Can you work these out from the model? Positions are in its coordinate system, mm. Face numbers are marked on the shaded views. A direction names the side the tool comes from. Coordinates: 2 decimals unless noted, no trailing zeros. Order: outer loops, then holes, each group sorted by start corner. A loop starts at its lowest first (then second) coordinate and runs counter-clockwise, first axis right, second up. Notation, with made-up numbers: M 63,69 L 83,69 A10 ccw 83,73 Z; hole C 43,42.25 d2. An arc over 180 degrees is marked long. Answer as a JSON object with one key per item and string values.
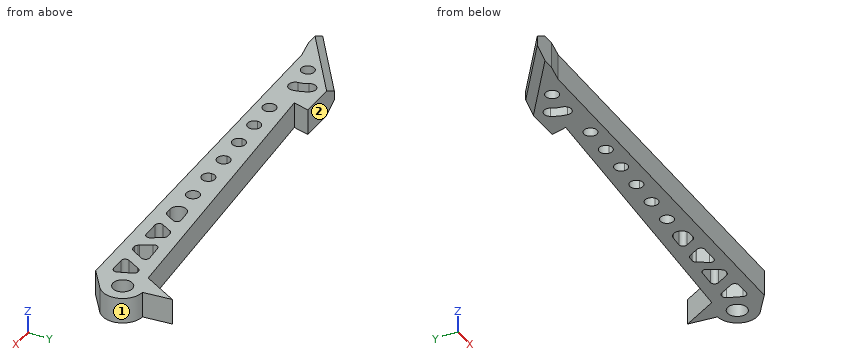
from build123d import *

# Parameters (mm, degrees)
SKETCH1_R           = 3.2639
SKETCH1_R_2         = 4.8025
BOSS_EXTRUDE1_DEPTH = 12.7
EXTRUDE_THIN1_DEPTH = 12.7
FILLET1_R           = 2
SKETCH3_R           = 3.2639
CUT_EXTRUDE1_DEPTH  = 222.669325799
CHAMFER1_SIZE       = 4


with BuildPart() as part:
    # Sketch1 → Boss-Extrude1 (new body)
    with BuildSketch(Plane.XY):
        with BuildLine():
            Line((-220, -20.475), (-207.3, -20.475))
            Line((-207.3, -20.475), (-197.3, -18.475))
            Line((-197.3, -18.475), (-5, -15.975))
            Line((-5, -15.975), (5.868885021, -8.096677628))
            ThreePointArc((5.868885021, -8.096677628), (9.584297561, 2.85328587), (0.484930071, 9.988235221))
            Line((0.484930071, 9.988235221), (-0.740940503, 24))
            Line((-0.740940503, 24), (-10.691733631, 6.764720727))
            Line((-10.691733631, 6.764720727), (-162.296299831, -3.282137227))
            Line((-162.296299831, -3.282137227), (-160.296299831, 4.525))
            Line((-160.296299831, 4.525), (-184.296299831, 4.525))
            Line((-184.296299831, 4.525), (-220, -20.475))
        make_face()
        with Locations((-154, -10.975)):
            Circle(SKETCH1_R, mode=Mode.SUBTRACT)
        with BuildLine():
            ThreePointArc((-135.489653222, -10.110575335), (-138.597743308, -13.523178805), (-142.010346778, -10.415088719))
            ThreePointArc((-142.010346778, -10.415088719), (-138.902256692, -7.00248525), (-135.489653222, -10.110575335))
        make_face(mode=Mode.SUBTRACT)
        with BuildLine():
            ThreePointArc((-120.239653222, -9.398407362), (-123.347743308, -12.811010832), (-126.760346778, -9.702920746))
            ThreePointArc((-126.760346778, -9.702920746), (-123.652256692, -6.290317277), (-120.239653222, -9.398407362))
        make_face(mode=Mode.SUBTRACT)
        with BuildLine():
            ThreePointArc((-104.989653222, -8.686239389), (-108.097743308, -12.098842859), (-111.510346778, -8.990752773))
            ThreePointArc((-111.510346778, -8.990752773), (-108.402256692, -5.578149304), (-104.989653222, -8.686239389))
        make_face(mode=Mode.SUBTRACT)
        with BuildLine():
            ThreePointArc((-89.739653222, -7.974071416), (-92.847743308, -11.386674886), (-96.260346778, -8.2785848))
            ThreePointArc((-96.260346778, -8.2785848), (-93.152256692, -4.865981331), (-89.739653222, -7.974071416))
        make_face(mode=Mode.SUBTRACT)
        with Locations((-77.75, -7.414160135)):
            Circle(SKETCH1_R, mode=Mode.SUBTRACT)
        with BuildLine():
            ThreePointArc((-63.032372648, -10.728944003), (-67.081236547, -6.887586999), (-63.348870778, -2.738036629))
            Line((-63.348870778, -2.738036629), (-11.492502478, 0.698492886))
            Line((-11.492502478, 0.698492886), (-7.437965658, -10.006187802))
            Line((-7.437965658, -10.006187802), (-63.032372648, -10.728944003))
        make_face(mode=Mode.SUBTRACT)
        Circle(SKETCH1_R_2, mode=Mode.SUBTRACT)
    extrude(amount=BOSS_EXTRUDE1_DEPTH)

    # Sketch2 → Extrude-Thin1 (add)
    with BuildSketch(Plane.XY.offset(12.7)):
        Polygon((-18.82367626, 4.244152852), (-20.32367626, 1.646076641), (-26.38156986, -8.846502861), (-27.88156986, -11.444579073), (-23.11843014, -14.194579073), (-21.61843014, -11.596502861), (-15.560536539, -1.103923359), (-14.060536539, 1.494152852), align=None)
        Polygon((-29.564922949, -12.326360556), (-31.654014309, -8.915246766), (-37.279649193, 0.270412174), (-39.368740553, 3.681525964), (-44.059022015, 0.809025344), (-41.969930654, -2.602088446), (-36.34429577, -11.787747387), (-34.25520441, -15.198861177), align=None)
        Polygon((-51.506359784, 2.078266381), (-53.006359784, -0.51980983), (-58.05148802, -9.258228266), (-59.55148802, -11.856304478), (-54.7883483, -14.606304478), (-53.2883483, -12.008228266), (-48.243220063, -3.26980983), (-46.743220063, -0.671733619), align=None)
    extrude(amount=-EXTRUDE_THIN1_DEPTH)

    # Fillet1
    fillet1_edges = [part.edges().sort_by_distance(p)[0] for p in [
        (-37.198435549, -10.393089387, 6.35),
        (-42.723767146, -1.371207834, 6.35),
        (-30.79987453, -10.309904766, 6.35),
        (-36.525812701, -0.960468438, 6.35),
        (-58.869359177, -10.674822663, 6.35),
        (-53.926545163, -2.113617659, 6.35),
        (-52.470477143, -10.591633869, 6.35),
        (-47.323034685, -1.676002002, 6.35),
        (-7.437965658, -10.006187802, 6.35),
        (-11.492502478, 0.698492886, 6.35),
        (-14.640351161, 0.489884469, 6.35),
        (-21.243861639, 0.052268813, 6.35),
        (-27.199441017, -10.263097258, 6.35),
        (-20.800558983, -10.179908464, 6.35),
    ]]
    fillet(fillet1_edges, radius=FILLET1_R)

    # Sketch3 → Cut-Extrude1 (cut, through all)
    with BuildSketch(Plane.XY.offset(12.7)):
        with Locations((-188, -10.475)):
            Circle(SKETCH3_R)
        with BuildLine():
            ThreePointArc((-170.811018785, -8.85662125), (-171.599559812, -5.080022092), (-173.207049233, -1.57281866))
            ThreePointArc((-173.207049233, -1.57281866), (-177.688057419, -0.458809846), (-178.802066233, -4.939818032))
            ThreePointArc((-178.802066233, -4.939818032), (-177.802564412, -7.120520542), (-177.31226682, -9.468727432))
            ThreePointArc((-177.31226682, -9.468727432), (-173.755589711, -12.413298359), (-170.811018785, -8.85662125))
        make_face()
    extrude(amount=-CUT_EXTRUDE1_DEPTH, mode=Mode.SUBTRACT)

    # Chamfer1
    chamfer1_edges = [part.edges().sort_by_distance(p)[0] for p in [
        (-202.148149916, -7.975, 0),
        (-202.148149916, -7.975, 12.7),
    ]]
    chamfer(chamfer1_edges, length=CHAMFER1_SIZE)


solid = part.part
Item 1: Please list where these lines run through material, in increasing order: line 1 (Y direction, x = -188, z = 5.75); line 2 (Y direction, x = -154, z = 5.5); line 3 (Y direction, x = -205.5, z = 3) (3 decimals).
Answers follow:
{"line 1": "y = -18.35 to -13.74, -7.21 to 1.93", "line 2": "y = -17.91 to -14.24, -7.71 to -2.73", "line 3": "y = -20.115 to -11.543"}
Item 2: I want a section at B-B, the plane y = 14. Write out the boundary of the cut face in (x, z).
Answers follow:
{"outline": "M -6.51,0 L 0.13,0 L 0.13,12.7 L -6.51,12.7 Z"}
Item 3: I want a section at D-D, the plane z = 2. Give the number of separate pieces and of enclosed holes in the cut face, plus the area to 3 significant figures.
Answers follow:
{"separate pieces": "1", "enclosed holes": "13", "area": "3,460 mm^2"}
Item 4: I'm going to push flat-ended pins straight in: pin 1 (12.5 mm diameter, centred on x = 0, y = 0, fed in from +Z); pin 2 (1 mm diameter, centred on y = 15, z = 8.5, fed in from -X); pin 3 (3 mm diameter, centred on y = 15.5, z = 6, fed in from -X); pin 4 (5 mm diameter, centred on y = 3.5, z = 3, fed in from +X). Where does each tip first touch, or does it pass through?
Answers follow:
{"pin 1": "stops at z = 12.7", "pin 2": "stops at x = -6.23", "pin 3": "stops at x = -6.51", "pin 4": "stops at x = 9.95"}
Item 5: Which directions (+Z, -Z, +X, -X, +Y, -Y) give clear straight access to the entire face, cutting with the end or side of a thin tool? Please do the marked faces 1 and 2.
Answers follow:
{"face 1": "+Z, -Z, +X", "face 2": "+Z, -Z, -X, +Y"}
Item 6: I want a section at A-A, the plane x = -188. Write out the boundary of the cut face in (y, z), plus the area to 3 significant figures.
Answers follow:
{"outline": "M -18.35,0 L -13.74,0 L -13.74,12.7 L -18.35,12.7 Z; M -7.21,0 L -2.95,0 L 1.93,4 L 1.93,8.7 L -2.95,12.7 L -7.21,12.7 Z", "area": "155 mm^2"}
Item 7: I want a section at C-C, the plane x = -108.25. Write out the boundary of the cut face in (y, z).
Answers follow:
{"outline": "M -17.32,0 L -12.1,0 L -12.1,12.7 L -17.32,12.7 Z; M -5.57,0 L 0.3,0 L 0.3,12.7 L -5.57,12.7 Z"}
